```python
from build123d import *

# Parameters (mm, degrees)
BOSS_EXTRUDE1_DEPTH      = 75.75
CUT_EXTRUDE1_DEPTH       = 144.384624803
BOSS_EXTRUDE2_DEPTH      = 10
BOSS_EXTRUDE2_DEPTH_BACK = 73.12
SKETCH3_R                = 4.9
SKETCH4_R                = 5
CUT_EXTRUDE2_DEPTH       = 10
SKETCH5_W                = 2
SKETCH5_H                = 13.39
CUT_EXTRUDE3_DEPTH       = 137.266849467
SKETCH6_W                = 10
SKETCH6_H                = 2
CUT_EXTRUDE4_DEPTH       = 137.266849467


with BuildPart() as part:
    # Sketch1 → Boss-Extrude1 (new body)
    with BuildSketch(Plane(origin=(0, 0, 0), x_dir=(0, 0, -1), z_dir=(1, 0, 0))):
        Polygon((-39.615373705, 97.524665991), (15.504626295, 97.524665991), (25.254562849, 97.524665991), (25.254562849, 84.134665991), (15.504626295, 77.134665991), (15.504626295, -72.475334009), (-47.615373705, -72.475334009), (-47.615373705, 84.134665991), (-39.615373705, 84.134665991), align=None)
    extrude(amount=BOSS_EXTRUDE1_DEPTH)

    # Sketch2 → Cut-Extrude1 (cut, through all)
    with BuildSketch(Plane.XY.offset(47.615373705)):
        Polygon((0, -59.755334009), (14.83, -72.475334009), (0, -72.475334009), align=None)
        Polygon((75.75, -59.755334009), (60.92, -72.475334009), (75.75, -72.475334009), align=None)
    extrude(amount=-CUT_EXTRUDE1_DEPTH, mode=Mode.SUBTRACT)

    # Sketch3 → Boss-Extrude2 (add, two sides: drawn at the far end of the back side and taken through both)
    with BuildSketch(Plane.XY.offset(47.615373705).offset(-BOSS_EXTRUDE2_DEPTH_BACK)):
        with Locations((37.875, -58.705334009)):
            Circle(SKETCH3_R)
    extrude(amount=BOSS_EXTRUDE2_DEPTH + BOSS_EXTRUDE2_DEPTH_BACK)

    # Sketch4 → Cut-Extrude2 (cut)
    with BuildSketch(Plane(origin=(0, 97.524665991, 0), x_dir=(1, 0, 0), z_dir=(0, 1, 0))):
        with Locations(Location((37.875, -7.180405428, 0), (0, 0, 270))):
            Circle(SKETCH4_R)
    extrude(amount=-CUT_EXTRUDE2_DEPTH, mode=Mode.SUBTRACT)

    # Sketch5 → Cut-Extrude3 (cut, through all)
    with BuildSketch(Plane(origin=(75.75, 0, 0), x_dir=(0, 0, -1), z_dir=(1, 0, 0))):
        with Locations((-38.615373705, 90.829665991)):
            Rectangle(SKETCH5_W, SKETCH5_H)
    extrude(amount=-CUT_EXTRUDE3_DEPTH, mode=Mode.SUBTRACT)

    # Sketch6 → Cut-Extrude4 (cut, through all)
    with BuildSketch(Plane(origin=(75.75, 0, 0), x_dir=(0, 0, -1), z_dir=(1, 0, 0))):
        with Locations((-42.615373705, 83.134665991)):
            Rectangle(SKETCH6_W, SKETCH6_H)
    extrude(amount=-CUT_EXTRUDE4_DEPTH, mode=Mode.SUBTRACT)


solid = part.part
```
Input: part model. Units: mm. Frame: model coordinates. A direction names the side the tool comes from. Coordinates: 2 decimals unless noted, no trailing zeros. Loops run counter-clockwise (first coordinate to the right, second up) from the corner with the lowest first, then second, coordinate; pieces in that order, holes last. Notation, with made-up numbers: M 9.5,-33 L 58.5,-33 A28 cw 58.5,-14 Z; hole C 80.5,77 d9. An arc over 180 degrees is marked long. Use a Markdown table: item, result. Add a question column.
1) Section D-D, the plane y = -41. Return the cut outline in (x, z), plus the area to 3 significant figures.
2) Pin query (flat end, axial travel): P1, Ø1, axis at x = 31.5, y = -7, coming from the +Z side; P2, Ø3, axis at x = 37.5, z = 8, coming from the +Y side; P3, Ø6.5, axis at x = 46.5, y = 93.5, coming from the -Z side. Return the tip coordinate at first contact, or that it passes through.
3) Set-up query: faces 1 (the cylindrical face through (42.832, 92.595, 6.53)), 2 (the flat face through (68.439, -66.026, 16.497)), 3 (the flat face through (38, 90, 37.615)). Return all of +Z, -Z, +X, -X, +Y, -Y with unobstructed straight access to the full face (end or side cutting, diameter ignored); none if empty.
4) Draft query along Y for faces 4 (the cylindrical face through (34.263, -55.394, -20.575)), 5 (the flat face through (38, 87.525, 7)), 6 (the cylindrical face through (34.263, -55.394, 52.545)). Return one class per face: +Y half, -Y half, draft (parallel to the pull), parting line (faces both ways), or undercut.
5) Section A-A, the plane z = 42. Return the cut outline in (x, y), plus the area to 3 significant figures.
6) Section B-B, the plane x = 16.5. Return the cut outline in (y, z).
7) Line query: L1, parallel to Z at x = 25.5, y = 71; L2, parallel to Y at x = 70.5, z = 18.5; L3, parallel to Y at x = 5.5, z = 16. Output: solid intervals per line, ascending. Write a range as from..to.
8) Section C-C, the plane z = -19. Return the cut outline in (x, y) (3 decimals), plus the area to 3 significant figures.
Answer below:
| question | item | result |
|---|---|---|
| 1 | outline | M 0,-15.5 L 75.75,-15.5 L 75.75,47.62 L 0,47.62 Z |
| 1 | area | 4,780 mm2 |
| 2 | P1 | z = 47.62 |
| 2 | P2 | y = 87.52 |
| 2 | P3 | z = -25.25 |
| 3 | face 1 | +Y |
| 3 | face 2 | +Z, -Z, +X, -Y |
| 3 | face 3 | +Z, +X, -X, +Y |
| 4 | face 4 | undercut |
| 4 | face 5 | +Y half |
| 4 | face 6 | parting line |
| 5 | outline | M 0,-59.76 L 14.83,-72.48 L 60.92,-72.48 L 75.75,-59.76 L 75.75,82.13 L 0,82.13 Z |
| 5 | area | 11,500 mm2 |
| 6 | outline | M -72.48,-15.5 L 77.13,-15.5 L 84.13,-25.25 L 97.52,-25.25 L 97.52,37.62 L 82.13,37.62 L 82.13,47.62 L -72.48,47.62 Z |
| 7 | L1 | -15.5..47.62 |
| 7 | L2 | -64.26..97.52 |
| 7 | L3 | -64.47..97.52 |
| 8 | outline | M 0,79.644 L 75.75,79.644 L 75.75,97.525 L 0,97.525 Z; C 37.875,-58.705 d9.8 |
| 8 | area | 1,430 mm2 |
